from build123d import *

# Parameters (mm, degrees)
FILLET1_R = 2.54


with BuildPart() as part:
    # Sketch1 → Revolve1 (revolve)
    with BuildSketch(Plane.XY, mode=Mode.PRIVATE) as revolve1_sk:
        Polygon((29.21, 0), (29.21, 19.05), (36.83, 19.05), (36.83, 17.78), (30.48, 17.78), (30.48, 0), align=None)
    revolve(revolve1_sk.sketch.rotate(Axis((0, 0, 0), (0, 1, 0)), 90), axis=Axis((0, 0, 0), (0, 1, 0)))

    # Fillet1
    fillet1_edges = [part.edges().sort_by_distance(p)[0] for p in [
        (0, 19.05, 29.21),
    ]]
    fillet(fillet1_edges, radius=FILLET1_R)


solid = part.part
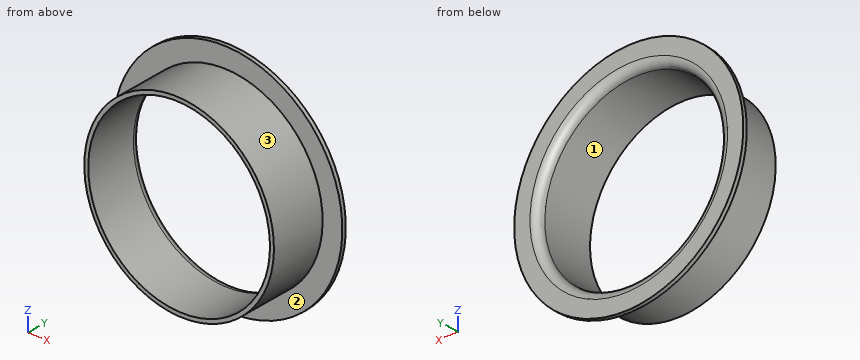
Can you work these out from the model? Positions are in its coordinate system, mm. Face numbers are marked on the shaded views. Coordinates: 2 decimals unless noted, no trailing zeros. Order: outer loops, then holes, each group sorted by start corner. A loop starts at its lowest first (then second) coordinate and runs counter-clockwise, first axis right, second up. Notation, with made-up numbers: M 54.5,54.5 L 113.5,54.5 A8 ccw 113.5,60.5 Z; hole C 15.5,8.25 d6. An arc over 180 degrees is marked long. Write item = value, one per line.
(1) I need wall thicknesses on line 1 along X through (y, z) = (6, 0); line 2 along X through (y, z) = (14, 2); line 3 along Z through (x, y) = (12, 16.75). Which ranges of each line are inside material? Lowest first, please. Write a range as [from, to].
Results are:
line_1 = [-30.48, -29.21], [29.21, 30.48]
line_2 = [-30.41, -29.14], [29.14, 30.41]
line_3 = [-28.02, -26.64], [26.64, 28.02]
(2) Suppose I cut it at B-B on z = 0. Please give me the cut outline in (x, y).
Results are:
outline = M -36.83,17.78 L -30.48,17.78 L -30.48,0 L -29.21,0 L -29.21,16.51 A2.54 ccw -31.75,19.05 L -36.83,19.05 Z; M 29.21,0 L 30.48,0 L 30.48,17.78 L 36.83,17.78 L 36.83,19.05 L 31.75,19.05 A2.54 ccw 29.21,16.51 Z
(3) Suppose I cut it at A-A on x = 0. Please give me the cut outline in (y, z), plus the area to 3 significant figures.
Results are:
outline = M 0,-30.48 L 17.78,-30.48 L 17.78,-36.83 L 19.05,-36.83 L 19.05,-31.75 A2.54 ccw 16.51,-29.21 L 0,-29.21 Z; M 0,29.21 L 16.51,29.21 A2.54 ccw 19.05,31.75 L 19.05,36.83 L 17.78,36.83 L 17.78,30.48 L 0,30.48 Z
area = 61.7 mm2
(4) Suppose I cut it at C-C on y = 5.5. Please give me the cut outline in (x, z).
Results are:
outline = C 0,0 d60.96; hole C 0,0 d58.42
(5) For pin 1 Ø5 at (x, z) = (-17.5, -24.5) entering from -Y; pin 2 Ø3 at (x, y) = (-3.5, 5.5) entering from -Z; pin 3 Ø1.5 at (x, y) = (-13.5, 11) entering from -Z; pin 4 Ø8 at (x, y) = (22.5, 3.5) entering from +Z, each with a flat end and sliding along its axis, tell me the tip position at first contact or that it passes through.
Results are:
pin_1 = 0
pin_2 = -30.41
pin_3 = -27.69
pin_4 = 24.22
(6) If we mould it in two halves opening along Z, with no side actions, what happens to the marked faces 1, 2 and 3? For each: pulls with the +Z half, pulls with the -Z half, needs draft (parallel to the pull), parting line crosses it, or undercut.
Results are:
face_1 = undercut
face_2 = needs draft
face_3 = parting line crosses it
